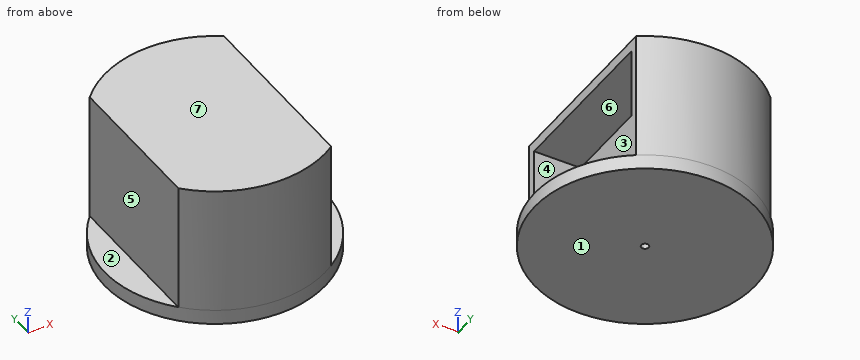
```python
from build123d import *

# Parameters (mm, degrees)
ESQUISSE1_R             = 30
BOSS_EXTRU_1_DEPTH      = 4
BOSS_EXTRU_3_DEPTH      = 35
ESQUISSE7_W             = 19
ESQUISSE7_H             = 45
ENL_V_MAT_EXTRU_1_DEPTH = 30
ESQUISSE8_R             = 1.001210448
ENL_V_MAT_EXTRU_2_DEPTH = 2


with BuildPart() as part:
    # Esquisse1 → Boss.-Extru.1 (new body)
    with BuildSketch(Plane.XY):
        with Locations((-21.677103804, 21.48828033)):
            Circle(ESQUISSE1_R)
    extrude(amount=BOSS_EXTRU_1_DEPTH)

    # Esquisse4 → Boss.-Extru.3 (add)
    with BuildSketch(Plane.XY.offset(4)):
        with BuildLine():
            Line((-43.677103804, 41.884358384), (-43.677103804, 21.48828033))
            Line((-43.677103804, 21.48828033), (-43.677103804, 1.092202275))
            ThreePointArc((-43.677103804, 1.092202275), (-24.981744089, -8.329153372), (-4.677103804, -3.230133859))
            Line((-4.677103804, -3.230133859), (-4.677103804, 46.206694518))
            ThreePointArc((-4.677103804, 46.206694518), (-24.981744089, 51.305714032), (-43.677103804, 41.884358384))
        make_face()
    extrude(amount=BOSS_EXTRU_3_DEPTH)

    # Esquisse7 → Enlèv. mat.-Extru.1 (cut)
    with BuildSketch(Plane(origin=(-4.677103804, 0, 0), x_dir=(0, 0, -1), z_dir=(1, 0, 0))):
        with Locations((-26.5, 21.706694518)):
            Rectangle(ESQUISSE7_W, ESQUISSE7_H)
    extrude(amount=-ENL_V_MAT_EXTRU_1_DEPTH, mode=Mode.SUBTRACT)

    # Esquisse8 → Enlèv. mat.-Extru.2 (cut)
    with BuildSketch(Plane(origin=(0, 0, 0), x_dir=(-1, 0, 0), z_dir=(0, 0, -1))):
        with Locations((21.677103804, 21.48828033)):
            Circle(ESQUISSE8_R)
    extrude(amount=-ENL_V_MAT_EXTRU_2_DEPTH, mode=Mode.SUBTRACT)


solid = part.part
```
Can you work these out from the model? Positions are in its coordinate system, mm. Face numbers are marked on the shaded views. A direction names the side the tool comes from. Coordinates: 2 decimals unless noted, no trailing zeros. Loops run counter-clockwise (first coordinate to the right, second up) from the corner with the lowest first, then second, coordinate; pieces in that order, holes last. Notation, with made-up numbers: (14.5, -26) -> (70.5, -26) arc R18 cw to (70.5, 0) -> close; hole circle Ø6 at (85, 63). An arc over 180 degrees is marked (long way). Put each result on its own line as item: value. Start each with the question number.
Q1. Thinking about a two-plate mould opening in Z: for the marked faces 5, 6 and 7, which applies, pulls with the +Z half, pulls with the -Z half, needs draft (parallel to the pull), parting line crosses it, or undercut?
Q2. I'm going to push flat-ended pins straight in: P1, Ø8, axis at y = 10.5, z = 24, coming from the +X side; P2, Ø6, axis at x = -28, z = 8.5, coming from the +Y side; P3, Ø5, axis at y = 40, z = 8.5, coming from the -X side. Where does each tip first touch, or does it pass through?
Q3. I want a section at B-B (z = 29). Write out the boundary of the cut face in (x, y), plus the area to 3 significant figures.
Q4. I want a section at C-C (y = 27). Write out the boundary of the cut face in (x, z), plus the area to 3 significant figures.
Q5. If I drill on line 1 (Z direction, x = -22.5, y = 16); line 2 (X direction, y = 10.5, z = 32.5); line 3 (Z direction, x = -45, y = 17), over which ranges is the centre line in solid material (lowest first)? Write a range as [from, to].
Q6. I want a section at D-D (x = -17.5). Write out the boundary of the cut face in (y, z).
Q7. For the marked faces 1, 2, 3 and 4, which set-ups out of +Z, -Z, +X, -X, +Y, -Y let a thin tool reach every point of the face, with its end or its side?
Q8. I want a section at A-A (x = -10). Write out the boundary of the cut face in (y, z), plus the area to 3 significant figures.
Taken from the geometry:
1. face 5: needs draft
1. face 6: undercut
1. face 7: pulls with the +Z half
2. P1: stops at x = -34.68
2. P2: stops at y = 51.3
2. P3: stops at x = -43.68
3. outline: (-43.68, 1.09) arc R30 ccw to (-4.68, -3.23) -> (-4.68, -0.79) -> (-34.68, -0.79) -> (-34.68, 44.21) -> (-4.68, 44.21) -> (-4.68, 46.21) arc R30 ccw to (-43.68, 41.88) -> close
3. area: 802 mm2
4. outline: (-51.17, 0) -> (7.81, 0) -> (7.81, 4) -> (-4.68, 4) -> (-4.68, 17) -> (-34.68, 17) -> (-34.68, 36) -> (-4.68, 36) -> (-4.68, 39) -> (-43.68, 39) -> (-43.68, 4) -> (-51.17, 4) -> close
4. area: 1,030 mm2
5. line 1: z = [0, 17], [36, 39]
5. line 2: x = [-43.68, -34.68]
5. line 3: z = [0, 4]
6. outline: (-8.22, 0) -> (51.2, 0) -> (51.2, 39) -> (-8.22, 39) -> close; hole (-0.79, 17) -> (44.21, 17) -> (44.21, 36) -> (-0.79, 36) -> close
7. face 1: -Z, +X, -X, +Y, -Y
7. face 2: +Z, -X, +Y, -Y
7. face 3: +Z, +X, +Y, -Y
7. face 4: +X
8. outline: (-6.15, 0) -> (49.12, 0) -> (49.12, 39) -> (-6.15, 39) -> close; hole (-0.79, 17) -> (44.21, 17) -> (44.21, 36) -> (-0.79, 36) -> close
8. area: 1,300 mm2
